Build history of the part. All positions in model axes, mm. A direction names the side the tool comes from. Round coordinates to 2 decimals unless told otherwise and drop trailing zeros. Write each loop counter-clockwise with the first axis right and the second up, starting at its lowest first coordinate (ties: lowest second). Pieces come first, ordered by that corner, then holes.
1) Flat gauge pins, fed straight in: pin 1 (10 mm diameter, centred on x = -17, z = 11.5, fed in from -Y); pin 2 (5 mm diameter, centred on x = 15, z = 27, fed in from +Y); pin 3 (11 mm diameter, centred on x = 11, z = 42.5, fed in from +Y). Where does each tip first touch, or does it go through?
2) Saw through at D-D (x = -11). Write the cut outline in (y, z), plus the area to 3 significant figures.
3) Wall check: probe 1 along Z at (x, y) = (-11, -6); probe 2 along Y at (x, z) = (10.5, 0.5); probe 3 along Z at (x, y) = (1.5, 75). Give the ranges that are in metal, low to high.
4) Saw through at C-C (z = 0). Write the cut outline in (x, y).
5) Which spindle directions (+Z, -Z, +X, -X, +Y, -Y) get a long thin tool onto all of the face, cutting with end or side? Do faces 1 (the flat face through (-11, 0, -42)), 2 (the flat face through (0, -12, 22.5)), 3 (the flat face through (0, -25, 38)). Say none if no direction does.
6) Pull direction X, two halves, no side cores. Call faces 4 (the cylindrical face through (-19.57, -12.68, 24)), 5 (the flat face through (-11, 0, 43)), 6 (the cylindrical face through (-11, -12, 46)), 7 (the flat face through (0, 26, -52.5)): +X half, -X half, draft (parallel to the pull), parting line (faces both ways), or undercut.
7) Saw through at A-A (y = -14.5). Write the cut outline in (x, z).
8) Saw through at B-B (x = -2.5). Write the cut outline in (y, z).
Autodesk Inventor part; units mm, degrees
ref_plane "YZ Plane" through (0, 0, 0) normal (1, 0, 0) x (0, 1, 0)
ref_plane "XZ Plane" through (0, 0, 0) normal (0, 1, 0) x (-1, 0, 0)
ref_plane "XY Plane" through (0, 0, 0) normal (0, 0, 1) x (1, 0, 0)
sketch "Sketch1" plane through (0, 0, 0) normal (0, 1, 0) x (-1, 0, 0)
  line L0 (-21, -52.5) -> (21, -52.5)
  line L1 (21, -52.5) -> (21, 52.5)
  line L2 (21, 52.5) -> (-21, 52.5)
  line L3 (-21, 52.5) -> (-21, -52.5)
  line L4 (-21, -52.5) -> (21, 52.5) construction
  line L5 (21, -52.5) -> (-21, 52.5) construction
  line L6 (-11, -42.5) -> (11, -42.5) construction
  line L7 (11, -42.5) -> (11, 42.5) construction
  line L8 (11, 42.5) -> (-11, 42.5) construction
  line L9 (-11, 42.5) -> (-11, -42.5) construction
  line L10 (-11, -42.5) -> (11, 42.5) construction
  line L11 (11, -42.5) -> (-11, 42.5) construction
  line L12 (-21, -22.5) -> (21, -22.5)
  line L13 (21, -22.5) -> (21, 22.5)
  line L14 (21, 22.5) -> (-21, 22.5)
  line L15 (-21, 22.5) -> (-21, -22.5)
  line L16 (-21, -22.5) -> (21, 22.5) construction
  line L17 (21, -22.5) -> (-21, 22.5) construction
  circle A0 centre (11, 42.5) radius 3.5
  circle A1 centre (-11, 42.5) radius 3.5
  circle A2 centre (11, -42.5) radius 3.5
  circle A3 centre (-11, -42.5) radius 3.5
  point P0 (0, 0)
  dimension "d0" = 22
  dimension "d1" = 85
  dimension "d2" = 10
  dimension "d3" = 10
  dimension "d4" = 45
  dimension "d5" = 7
  dimension "d6" = 7
  dimension "d8" = 7
  dimension "d9" = 7
extrude "Extrusion1" add sketch "Sketch1" against normal blind 25 contours L3 L12 L1 L0 | L3 L2 L1 L14
extrude "Extrusion2" add sketch "Sketch1" along normal blind 105 contours L3 L12 L1 L0 | L3 L14 L1 L12 | L3 L2 L1 L14 | A0 | A1 | A2 | A3
sketch "Sketch2" plane through (21, -25, -22.5) normal (1, 0, 0) x (0, 0, -1)
  circle A0 centre (-22.5, 91) radius 12.5
  line L0 (-45, 0) -> (-75, 0)
  line L1 (-22.5, 25) -> (-22.5, 91) construction
  dimension "d14" = 25
  dimension "d15" = 91
extrude "Extrusion3" cut sketch "Sketch2" against normal through all
fillet "Fillet1" radius 30 2 edges at (0, 105, 52.5) (0, 105, -52.5)
fillet "Fillet2" radius 5 14 edges at (21, 96.2132, 43.7132) (21, 105, 0) (21, 96.2132, -43.7132) (21, 25, -52.5) (21, 25, 52.5) (-21, 25, 52.5) (-21, 105, 0) (-21, 96.2132, -43.7132) (-21, 25, -52.5) (-21, 96.2132, 43.7132) (21, -12.5, 22.5) (21, -12.5, -22.5) (-21, -12.5, -22.5) (-21, -12.5, 22.5)
chamfer "Chamfer1" distance 4 angle 45 2 edges at (21, 66, 12.5) (-21, 66, 12.5)
equation "\"d3\" = d2"
equation "\"d6\" = d5"
equation "\"d8\" = d5"
equation "\"d9\" = d5"
properties part number "BALL SCREW MIDDLE SUPPORT"
Evaluation:
1. pin 1: stops at y = 0
1. pin 2: stops at y = 104.93
1. pin 3: stops at y = 101.26
2. outline: (-25, -52.5) - (75, -52.5) arc R30 ccw to (105, -22.5) - (105, 22.5) arc R30 ccw to (75, 52.5) - (-25, 52.5) - (-25, 46) - (0, 46) - (0, 39) - (-25, 39) - (-25, 22.5) - (0, 22.5) - (0, -22.5) - (-25, -22.5) - (-25, -39) - (0, -39) - (0, -46) - (-25, -46) - close; hole circle Ø25 at (66, 0)
2. area: 11,300 mm2
3. probe 1: z = -52.5 to -46, -39 to -22.5, 22.5 to 39, 46 to 52.5
3. probe 2: y = 0 to 53.51, 78.49 to 105
3. probe 3: z = -52.5 to -8.67, 8.67 to 52.5
4. outline: (-21, 0) - (21, 0) - (21, 49.5) - (17, 53.5) - (-17, 53.5) - (-21, 49.5) - close; (-21, 82.5) - (-17, 78.5) - (17, 78.5) - (21, 82.5) - (21, 100) arc R5 ccw to (16, 105) - (-16, 105) arc R5 ccw to (-21, 100) - close
5. face 1: -Y
5. face 2: +X, -X, -Y
5. face 3: +Z, -Z, +X, -X, -Y
6. face 4: -X half
6. face 5: undercut
6. face 6: undercut
6. face 7: draft
7. outline: (-21, -47.5) arc R5 ccw to (-16, -52.5) - (16, -52.5) arc R5 ccw to (21, -47.5) - (21, -27.5) arc R5 ccw to (16, -22.5) - (-16, -22.5) arc R5 ccw to (-21, -27.5) - close; (-21, 27.5) arc R5 ccw to (-16, 22.5) - (16, 22.5) arc R5 ccw to (21, 27.5) - (21, 47.5) arc R5 ccw to (16, 52.5) - (-16, 52.5) arc R5 ccw to (-21, 47.5) - close; hole circle Ø7 at (-11, -42.5); hole circle Ø7 at (-11, 42.5); hole circle Ø7 at (11, -42.5); hole circle Ø7 at (11, 42.5)
8. outline: (-25, -52.5) - (75, -52.5) arc R30 ccw to (105, -22.5) - (105, 22.5) arc R30 ccw to (75, 52.5) - (-25, 52.5) - (-25, 22.5) - (0, 22.5) - (0, -22.5) - (-25, -22.5) - close; hole circle Ø25 at (66, 0)
